from build123d import *

# Parameters (mm, degrees)
SKETCH1_W                                 = 146.05
SKETCH1_H                                 = 57.15
BOSS_EXTRUDE1_DEPTH                       = 3.175
F_6_CLEARANCE_HOLE1_D                     = 4.3053
F_1_2_0_5_DIAMETER_HOLE1_D                = 12.7
F_3_8_0_375_DIAMETER_HOLE1_D              = 9.525
F_1_8_0_125_DIAMETER_HOLE1_D              = 3.175
CSK_FOR_6_FLAT_HEAD_MACHINE_SCREW_2_COUNT = 2
CSK_FOR_6_FLAT_HEAD_MACHINE_SCREW_2_PITCH = 38.528341037
CSK_FOR_6_FLAT_HEAD_MACHINE_SCREW_3_COUNT = 2
CSK_FOR_6_FLAT_HEAD_MACHINE_SCREW_3_PITCH = 51.534810808
CSK_FOR_6_FLAT_HEAD_MACHINE_SCREW_4_COUNT = 2
CSK_FOR_6_FLAT_HEAD_MACHINE_SCREW_4_PITCH = 24.55


with BuildPart() as part:
    # Sketch1 → Boss-Extrude1 (new body)
    with BuildSketch(Plane.XY):
        with Locations((-73.025, 28.575)):
            Rectangle(SKETCH1_W, SKETCH1_H)
    extrude(amount=-BOSS_EXTRUDE1_DEPTH)

    # #6 Clearance Hole1 (through all)
    with Locations(Plane(origin=(0, 0, -3.175), x_dir=(-1, 0, 0), z_dir=(0, 0, -1))):
        with Locations((4.8895, 42.8625), (141.1605, 42.8625), (141.1605, 14.2875), (4.8895, 14.2875), (19.05, 47.752), (19.05, 9.398), (127, 9.398), (127, 47.752)):
            Hole(F_6_CLEARANCE_HOLE1_D / 2)

    # 1/2 (0.5) Diameter Hole1 (through all)
    with Locations(Plane(origin=(0, 0, -3.175), x_dir=(-1, 0, 0), z_dir=(0, 0, -1))):
        with Locations((76.2, 28.575), (120.65, 28.575)):
            Hole(F_1_2_0_5_DIAMETER_HOLE1_D / 2)

    # 3/8 (0.375) Diameter Hole1 (through all)
    with Locations(Plane(origin=(0, 0, -3.175), x_dir=(-1, 0, 0), z_dir=(0, 0, -1))):
        with Locations((31.75, 24.13)):
            Hole(F_3_8_0_375_DIAMETER_HOLE1_D / 2)

    # 1/8 (0.125) Diameter Hole1 (through all)
    with Locations(Plane(origin=(0, 0, -3.175), x_dir=(-1, 0, 0), z_dir=(0, 0, -1))):
        with Locations((76.2, 19.05)):
            Hole(F_1_8_0_125_DIAMETER_HOLE1_D / 2)

    # Sketch14 → CSK for #6 Flat Head Machine Screw (100)2 (revolve, cut)
    with BuildSketch(Plane(origin=(-63.5, 8.89, -3.175), x_dir=(0, 1, 0), z_dir=(1, 0, 0))):
        Polygon((0, 0), (0, 3.175), (2.15265, 3.175), (2.15265, 1.420893136), (3.8460045, 0), align=None)
    csk_for_6_flat_head_machine_screw_100 = revolve(axis=Axis((-63.5, 8.89, -9.525), (0, 0, 1)), mode=Mode.SUBTRACT)

    # CSK for _6 Flat Head Machine Screw _ 2: CSK for #6 Flat Head Machine Screw (100)2 ×2
    with Locations(*[Vector(0.217814006, 0.975990296, 0) * (i * CSK_FOR_6_FLAT_HEAD_MACHINE_SCREW_2_PITCH) for i in range(1, CSK_FOR_6_FLAT_HEAD_MACHINE_SCREW_2_COUNT)]):
        add(csk_for_6_flat_head_machine_screw_100, mode=Mode.SUBTRACT)

    # CSK for _6 Flat Head Machine Screw _ 3: CSK for #6 Flat Head Machine Screw (100)2 ×2
    with Locations(*[Vector(0.924132625, 0.38207184, 0) * (i * CSK_FOR_6_FLAT_HEAD_MACHINE_SCREW_3_PITCH) for i in range(1, CSK_FOR_6_FLAT_HEAD_MACHINE_SCREW_3_COUNT)]):
        add(csk_for_6_flat_head_machine_screw_100, mode=Mode.SUBTRACT)

    # CSK for _6 Flat Head Machine Screw _ 4: CSK for #6 Flat Head Machine Screw (100)2 ×2
    with Locations(*[(i * CSK_FOR_6_FLAT_HEAD_MACHINE_SCREW_4_PITCH, 0, 0) for i in range(1, CSK_FOR_6_FLAT_HEAD_MACHINE_SCREW_4_COUNT)]):
        add(csk_for_6_flat_head_machine_screw_100, mode=Mode.SUBTRACT)


solid = part.part
Part model, mm, in its own coordinate system. Give positions to 0.01 mm unless a question says otherwise; leave off trailing zeros. Put each result on its own line as item: value. Start each with the question number.
1) Pull direction Y, two halves, no side cores. Call faces 1 (the flat face through (-74, 35, -3.175)), 2 (the cylindrical face through (-56.563, 44.907, -0.889)), 3 (the flat face through (-74, 0, -2)): +Y half, -Y half, draft (parallel to the pull), parting line (faces both ways), or undercut.
2) Probe probe 1 along Y at (x, z) = (-19, -1.1); probe 2 along X at (y, z) = (14, -1.35); probe 3 along X at (y, z) = (27, -2). List the from-to ranges inside material, lowest first.
3) Saw through at B-B (x = -76.2). State how many separate pieces and enclosed holes the cut face has, then the cut area to 3 significant figures.
Numbers:
1. face 1: draft
1. face 2: undercut
1. face 3: -Y half
2. probe 1: 0 to 7.25, 11.55 to 45.6, 49.9 to 57.15
2. probe 2: -146.05 to -143.29, -139.03 to -7.02, -2.76 to 0
2. probe 3: -146.05 to -126.8, -114.5 to -82.35, -70.05 to -35.55, -27.95 to -17.74, -14.01 to 0
3. separate pieces: 3
3. enclosed holes: 0
3. area: 131 mm^2
